Work out the finished part from the listing and answer in its coordinate system (mm). Face numbers are marked on the shaded views. Round coordinates to 2 decimals unless told otherwise and drop trailing zeros. Write each loop counter-clockwise with the first axis right and the second up, starting at its lowest first coordinate (ties: lowest second). Pieces come first, ordered by that corner, then holes. Notation, with made-up numbers: (-27, -9) - (1, -9) arc R10 cw to (1, -4) - close; hole circle Ø9 at (37, 9.5). An arc over 180 degrees is marked (long way). Write item = value, one per line. Start each with the question number.
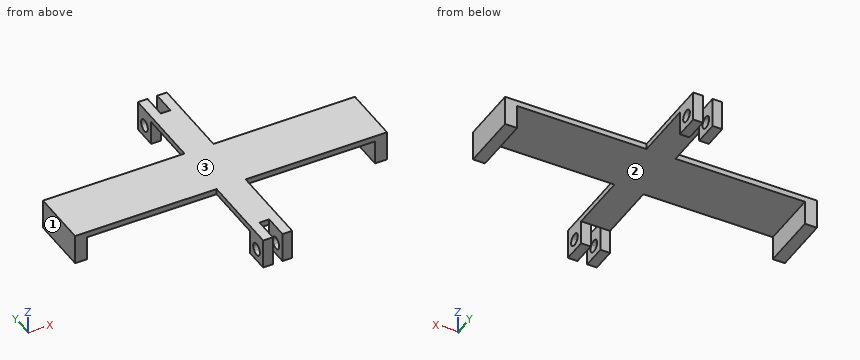
from build123d import *

# Parameters (mm, degrees)
F1_DEPTH = 3
F2_W     = 5.08
F2_H     = 12.7
F2_W_2   = 6.35
F2_H_2   = 30.7130107253
F3_DEPTH = 12.7
F4_R     = 3.175
F5_DEPTH = 25.4


with BuildPart() as f1:
    # F0 (on Top) → F1 (new body)
    with BuildSketch(Plane.XY):
        Polygon((-2.54, 59.944), (-7.62, 59.944), (-7.62, 15.3565053627), (-81.915, 15.3565053627), (-81.915, -15.3565053627), (-7.62, -15.3565053627), (-7.62, -59.944), (-2.54, -59.944), (-2.54, -53.594), (-2.54, -47.244), (2.54, -47.244), (2.54, -59.944), (2.8766005316, -59.944), (6.35, -59.944), (7.62, -59.944), (7.62, -15.3565053627), (81.915, -15.3565053627), (81.915, 15.3565053627), (7.62, 15.3565053627), (7.62, 59.944), (6.35, 59.944), (2.8766005316, 59.944), (2.54, 59.944), (2.54, 47.244), (-2.54, 47.244), (-2.54, 53.594), align=None)
    extrude(amount=F1_DEPTH)

    # F2 (on face) → F3 (join)
    with BuildSketch(Plane(origin=(0, 0, 0), x_dir=(1, 0, 0), z_dir=(0, 0, -1))):
        with Locations((-5.08, 53.594)):
            Rectangle(F2_W, F2_H)
        with Locations((5.08, 53.594)):
            Rectangle(F2_W, F2_H)
        with Locations((78.74, 0)):
            Rectangle(F2_W_2, F2_H_2)
        with Locations((5.08, -53.594)):
            Rectangle(F2_W, F2_H)
        with Locations((-5.08, -53.594)):
            Rectangle(F2_W, F2_H)
        with Locations((-78.74, 0)):
            Rectangle(F2_W_2, F2_H_2)
    extrude(amount=F3_DEPTH)

    # F4 (on face) → F5 (cut)
    with BuildSketch(Plane.YZ.offset(7.62)):
        with Locations((53.594, -6.35)):
            Circle(F4_R)
        with BuildLine():
            Line((-55.8390640303, -4.1049359697), (-51.3489359697, -8.5950640303))
            ThreePointArc((-51.3489359697, -8.5950640303), (-50.6606824843, -7.5650198978), (-50.419, -6.35))
            ThreePointArc((-50.419, -6.35), (-52.3789801022, -3.4166824843), (-55.8390640303, -4.1049359697))
        make_face()
        with BuildLine():
            ThreePointArc((-55.8390640303, -4.1049359697), (-55.8390640303, -8.5950640303), (-51.3489359697, -8.5950640303))
            Line((-51.3489359697, -8.5950640303), (-55.8390640303, -4.1049359697))
        make_face()
    extrude(amount=-F5_DEPTH, mode=Mode.SUBTRACT)


solid = f1.part
1. Find section A-A on y = -5. Give the vertices of the cut face in (x, z) (3 decimals), plus the area to 3 significant figures.
2. Find section B-B on x = 10. Give the vertices of the cut face in (y, z).
3. Find section C-C on y = -30. Give the vertices of the cut face in (x, z).
4. Consider line 1 (X direction, y = -9.5, z = -7.5) (3 decimals); line 2 (Z direction, x = 29, y = 9); line 3 (X direction, y = -34, z = 0.75). Determine where each line is inside the solid, lowest interval first.
5. Each of these flat-tipped pins is pushed along its axis until it touches: pin 1 (6 mm diameter, centred on x = 52, z = -2, fed in from -Y); pin 2 (8.5 mm diameter, centred on y = 53.594, z = -6.35, fed in from -X); pin 3 (4.5 mm diameter, centred on y = -36.5, z = -2.5, fed in from -X); pin 4 (5 mm diameter, centred on x = -59, y = -2, fed in from -Z). Where does it stop, or does it pass through?
6. For a pull along Z with two mould halves and no side action, classify the marked faces 1, 2 and 3 as released by +Z, released by -Z, zero draft, split by the parting line, or undercut.
Answer key:
q1.outline = (-81.915, -12.7) - (-75.565, -12.7) - (-75.565, 0) - (75.565, 0) - (75.565, -12.7) - (81.915, -12.7) - (81.915, 3) - (-81.915, 3) - close
q1.area = 653 mm²
q2.outline = (-15.36, 0) - (15.36, 0) - (15.36, 3) - (-15.36, 3) - close
q3.outline = (-7.62, 0) - (7.62, 0) - (7.62, 3) - (-7.62, 3) - close
q4.line_1 = -81.915 to -75.565, 75.565 to 81.915
q4.line_2 = 0 to 3
q4.line_3 = -7.62 to 7.62
q5.pin_1 = -15.36
q5.pin_2 = -7.62
q5.pin_3 = through
q5.pin_4 = 0
q6.face_1 = zero draft
q6.face_2 = released by -Z
q6.face_3 = released by +Z
